```python
from build123d import *

# Parameters (mm, degrees)
FILLET1_R = 0.1


with BuildPart() as part:
    # Sketch1 → Revolve1 (revolve)
    with BuildSketch(Plane(origin=(0, 0, 0), x_dir=(0, 0, -1), z_dir=(1, 0, 0)), mode=Mode.PRIVATE) as revolve1_sk:
        Polygon((-2.1, 5), (-2.1, 5.4), (-2, 5.4), (-2, 6.95), (-2.1, 6.95), (-2.1, 7.35), (2.1, 7.35), (2.1, 6.95), (2, 6.95), (2, 5.4), (2.1, 5.4), (2.1, 5), align=None)
    revolve(revolve1_sk.sketch.rotate(Axis((0, 0, 14.88), (0, 0, -1)), 90), axis=Axis((0, 0, 14.88), (0, 0, -1)))

    # Fillet1
    fillet1_edges = [part.edges().sort_by_distance(p)[0] for p in [
        (-7.35, 0, 2.1),
        (-7.35, 0, -2.1),
        (-5, 0, -2.1),
        (-5, 0, 2.1),
    ]]
    fillet(fillet1_edges, radius=FILLET1_R)


solid = part.part
```
Here's how the part is built. I have some questions about the finished solid (model axes, mm). Coordinates: 2 decimals unless noted, no trailing zeros. Order: outer loops, then holes, each group sorted by start corner. A loop starts at its lowest first (then second) coordinate and runs counter-clockwise, first axis right, second up. Notation, with made-up numbers: M 17,44 L 59,44 A23 cw 59,54 Z; hole C 5.5,-24 d8. An arc over 180 degrees is marked long. Answer as a JSON object with one key per item and string values. Group by question number.
(1) Suppose I cut it at C-C, the plane z = 0.65. Please give me the cut outline in (x, y).
(2) I need wall thicknesses on probe 1 along Y at (x, z) = (0, -1.95); probe 2 along Z at (x, y) = (-4.5, -4); probe 3 along Y at (x, z) = (-2.5, 0.7). Which ranges of each line are inside material? Lowest first, please.
(3) For pin 1 (1 mm diameter, centred on y = 3, z = -0.5, fed in from -X); pin 2 (1.5 mm diameter, centred on x = -3.5, z = 1, fed in from +Y), each with a flat end and sliding along its axis, tell me the tip position at first contact or that it passes through.
(4) If we mould it in two halves opening along X, with no side actions, what happens to faces 1 (the face through (-5, 0, 0)), 2 (the face through (-4, 4, 2)), 3 (the face through (-1.593, 7.175, -0.028))? For each: released by +X, released by -X, zero draft, split by the parting line, or undercut.
Values found:
{
 "1": {"outline": "C 0,0 d14.7; hole C 0,0 d10"},
 "2": {"probe 1": "y = -7.35 to -5, 5 to 7.35", "probe 2": "z = -2 to 2", "probe 3": "y = -6.91 to -4.33, 4.33 to 6.91"},
 "3": {"pin 1": "stops at x = -6.91", "pin 2": "stops at y = 6.82"},
 "4": {"face 1": "undercut", "face 2": "undercut", "face 3": "split by the parting line"}
}
